Read the model definition and answer for the solid it produces. Units are mm, in the model's axes. Coordinates: 2 decimals unless noted, no trailing zeros. Write each loop counter-clockwise with the first axis right and the second up, starting at its lowest first coordinate (ties: lowest second). Pieces come first, ordered by that corner, then holes. Notation, with made-up numbers: (82, -22) -> (125, -22) arc R29 ccw to (125, 8) -> close; hole circle Ø4 at (-11.75, -25). An arc over 180 degrees is marked (long way). Use CSV: the item, a comma, the result in double quotes. Start each with the question number.
from build123d import *

# Parameters (mm, degrees)
F0_W     = 177.8
F0_H     = 76.2
F0_R     = 2.3876
F1_DEPTH = 12.7
F3_DEPTH = 5.207
F5_D     = 4.7752
F5_DEPTH = 19.05
F5_TIP   = 1.434614814


with BuildPart() as f1:
    # F0 (on Top) → F1 (new body)
    with BuildSketch(Plane.XY):
        with Locations((26.67, -19.6088)):
            Rectangle(F0_W, F0_H)
        with BuildLine():
            ThreePointArc((-48.895, -29.083), (-51.308, -26.67), (-48.895, -24.257))
            Line((-48.895, -24.257), (-42.545, -24.257))
            ThreePointArc((-42.545, -24.257), (-40.132, -26.67), (-42.545, -29.083))
            Line((-42.545, -29.083), (-48.895, -29.083))
        make_face(mode=Mode.SUBTRACT)
        with Locations((77.47, -45.0088)):
            Circle(F0_R, mode=Mode.SUBTRACT)
        with BuildLine():
            ThreePointArc((33.655, -29.083), (31.242, -26.67), (33.655, -24.257))
            Line((33.655, -24.257), (40.005, -24.257))
            ThreePointArc((40.005, -24.257), (42.418, -26.67), (40.005, -29.083))
            Line((40.005, -29.083), (33.655, -29.083))
        make_face(mode=Mode.SUBTRACT)
        with BuildLine():
            ThreePointArc((-48.895, -2.413), (-51.308, 0), (-48.895, 2.413))
            Line((-48.895, 2.413), (-42.545, 2.413))
            ThreePointArc((-42.545, 2.413), (-40.132, 0), (-42.545, -2.413))
            Line((-42.545, -2.413), (-48.895, -2.413))
        make_face(mode=Mode.SUBTRACT)
        with BuildLine():
            Line((40.005, -2.413), (33.655, -2.413))
            ThreePointArc((33.655, -2.413), (31.242, 0), (33.655, 2.413))
            Line((33.655, 2.413), (40.005, 2.413))
            ThreePointArc((40.005, 2.413), (42.418, 0), (40.005, -2.413))
        make_face(mode=Mode.SUBTRACT)
        with Locations((77.47, 5.7912)):
            Circle(F0_R, mode=Mode.SUBTRACT)
    extrude(amount=-F1_DEPTH)

    # F2 (on face) → F3 (cut)
    with BuildSketch(Plane.XY):
        with BuildLine():
            Line((-42.545, 3.9624), (-48.895, 3.9624))
            ThreePointArc((-48.895, 3.9624), (-52.8574, 0), (-48.895, -3.9624))
            Line((-48.895, -3.9624), (-42.545, -3.9624))
            ThreePointArc((-42.545, -3.9624), (-38.5826, 0), (-42.545, 3.9624))
        make_face()
        with BuildLine():
            Line((33.655, -3.9624), (40.005, -3.9624))
            ThreePointArc((40.005, -3.9624), (43.9674, 0), (40.005, 3.9624))
            Line((40.005, 3.9624), (33.655, 3.9624))
            ThreePointArc((33.655, 3.9624), (29.6926, 0), (33.655, -3.9624))
        make_face()
        with BuildLine():
            ThreePointArc((40.005, -30.6324), (43.9674, -26.67), (40.005, -22.7076))
            Line((40.005, -22.7076), (33.655, -22.7076))
            ThreePointArc((33.655, -22.7076), (29.6926, -26.67), (33.655, -30.6324))
            Line((33.655, -30.6324), (40.005, -30.6324))
        make_face()
        with BuildLine():
            Line((-42.545, -22.7076), (-48.895, -22.7076))
            ThreePointArc((-48.895, -22.7076), (-52.8574, -26.67), (-48.895, -30.6324))
            Line((-48.895, -30.6324), (-42.545, -30.6324))
            ThreePointArc((-42.545, -30.6324), (-38.5826, -26.67), (-42.545, -22.7076))
        make_face()
    extrude(amount=-F3_DEPTH, mode=Mode.SUBTRACT)

    # F5
    with Locations(Plane.YZ.offset(115.57)):
        with Locations((-48.1838, -6.35), (8.9662, -6.35)):
            Hole(F5_D / 2, depth=F5_DEPTH)
            with Locations((0, 0, -(F5_DEPTH + F5_TIP / 2))):  # 118° drill point
                Cone(0, F5_D / 2, F5_TIP, mode=Mode.SUBTRACT)


solid = f1.part
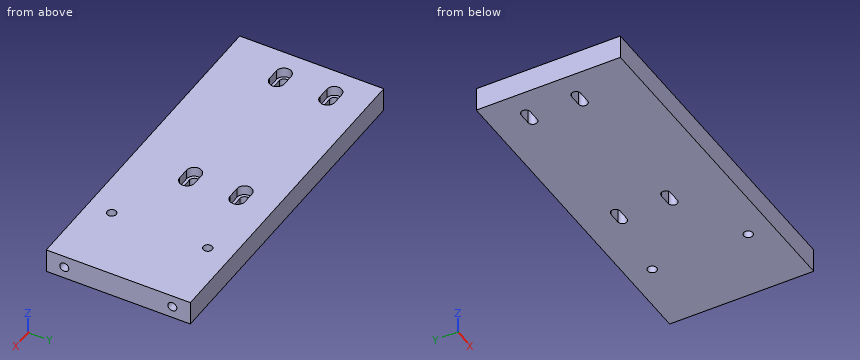
1) Section A-A, the plane y = 0 is taken. Give the vertices of the cut face in (x, z).
2) Section B-B, the plane x = 77.47 is taken. Give the vertices of the cut face in (y, z).
3) Find the intervals of material crossed by line 1 along Y through (x, z) = (77.47, -7.25); line 2 along Y through (x, z) = (110.25, -6.35); line 3 along X through (y, z) = (-25.5, -10.5), in increasing order.
4) Each of these flat-tipped pins is pushed along its axis until it touches: pin 1 (4.5 mm diameter, centred on y = 8.97, z = -6.35, fed in from +X); pin 2 (4 mm diameter, centred on x = 36, y = 0, fed in from +Z). Where does it stop, or does it pass through?
The answers:
1,outline,"(-62.23, -12.7) -> (-51.31, -12.7) -> (-51.31, -5.21) -> (-52.86, -5.21) -> (-52.86, 0) -> (-62.23, 0) -> close; (-40.13, -12.7) -> (31.24, -12.7) -> (31.24, -5.21) -> (29.69, -5.21) -> (29.69, 0) -> (-38.58, 0) -> (-38.58, -5.21) -> (-40.13, -5.21) -> close; (42.42, -12.7) -> (115.57, -12.7) -> (115.57, 0) -> (43.97, 0) -> (43.97, -5.21) -> (42.42, -5.21) -> close"
2,outline,"(-57.71, -12.7) -> (-47.4, -12.7) -> (-47.4, 0) -> (-57.71, 0) -> close; (-42.62, -12.7) -> (3.4, -12.7) -> (3.4, 0) -> (-42.62, 0) -> close; (8.18, -12.7) -> (18.49, -12.7) -> (18.49, 0) -> (8.18, 0) -> close"
3,line 1,"y = -57.71 to -47.4, -42.62 to 3.4, 8.18 to 18.49"
3,line 2,"y = -57.71 to -50.57, -45.8 to 6.58, 11.35 to 18.49"
3,line 3,"x = -62.23 to -51.01, -40.43 to 31.54, 42.12 to 115.57"
4,pin 1,"stops at x = 96.44"
4,pin 2,"passes through"
